from build123d import *

# Parameters (mm, degrees)
F0_W      = 39.5
F0_H      = 15
F1_DEPTH  = 5
F2_W      = 1.5
F2_H      = 15
F3_DEPTH  = 15
F5_W      = 1.5
F5_H      = 15
F6_DEPTH  = 15
F7_DEPTH  = 12.95
F9_W      = 0.5
F9_H      = 1.5
F10_DEPTH = 15
F9_W_2    = 1.5
F9_H_2    = 2.05
F9_H_3    = 2.0491243154
F11_DEPTH = 15
F13_DEPTH = 15
F14_W     = 0.5
F14_H     = 1.45
F15_DEPTH = 15


# Not quite as in the source:
# - the program builds the solid bodies; features that only make, move or delete a surface that nothing else refers to are left out


with BuildPart() as f1:
    # F0 (on Top) → F1 (new body)
    with BuildSketch(Plane.XY):
        Rectangle(F0_W, F0_H)
    extrude(amount=F1_DEPTH)

    # F2 (on face) → F3 (join)
    with BuildSketch(Plane.XY.offset(5)):
        with Locations((-19, 0)):
            Rectangle(F2_W, F2_H)
        with Locations((-9.5, 0)):
            Rectangle(F2_W, F2_H)
        Rectangle(F2_W, F2_H)
        with Locations((9.5, 0)):
            Rectangle(F2_W, F2_H)
        with Locations((19, 0)):
            Rectangle(F2_W, F2_H)
    extrude(amount=F3_DEPTH)

    # F5 (on face) → F6 (join)
    with BuildSketch(Plane(origin=(0, 0, 0), x_dir=(1, 0, 0), z_dir=(0, 0, -1))):
        with Locations((-19, 0)):
            Rectangle(F5_W, F5_H)
        with Locations((19, 0)):
            Rectangle(F5_W, F5_H)
    extrude(amount=F6_DEPTH)

    # F5 (on face) → F7 (join)
    with BuildSketch(Plane(origin=(0, 0, 0), x_dir=(1, 0, 0), z_dir=(0, 0, -1))):
        with Locations((-9.5, 0)):
            Rectangle(F5_W, F5_H)
        Rectangle(F5_W, F5_H)
        with Locations((9.5, 0)):
            Rectangle(F5_W, F5_H)
    extrude(amount=F7_DEPTH)

    # F9 (on face) → F10 (cut)
    with BuildSketch(Plane(origin=(0, 7.5, 0), x_dir=(-1, 0, 0), z_dir=(0, 1, 0))):
        with Locations((18.5, 18.75)):
            Rectangle(F9_W, F9_H)
        with Locations((-18.5, 18.75)):
            Rectangle(F9_W, F9_H)
    extrude(amount=-F10_DEPTH, mode=Mode.SUBTRACT)

    # F9 (on face) → F11 (cut)
    with BuildSketch(Plane(origin=(0, 7.5, 0), x_dir=(-1, 0, 0), z_dir=(0, 1, 0))):
        with Locations((-9.5, 18.975)):
            Rectangle(F9_W_2, F9_H_2)
        with Locations((0, 18.9754378423)):
            Rectangle(F9_W_2, F9_H_3)
        with Locations((9.5, 18.9754378423)):
            Rectangle(F9_W_2, F9_H_3)
    extrude(amount=-F11_DEPTH, mode=Mode.SUBTRACT)

    # F12 (on face) → F13 (join)
    with BuildSketch(Plane.XZ.offset(7.5)):
        Polygon((-18.25, 19.5), (-18.75, 19.5), (-18.75, 18.05), (18.7, 18.05), (18.7, 19.5), (18.25, 19.5), align=None)
    extrude(amount=-F13_DEPTH)

    # F14 (on face) → F15 (cut)
    with BuildSketch(Plane.XZ.offset(7.5)):
        with Locations((18.5, -13.775)):
            Rectangle(F14_W, F14_H)
        with Locations((-18.5, -13.775)):
            Rectangle(F14_W, F14_H)
    extrude(amount=-F15_DEPTH, mode=Mode.SUBTRACT)


solid = f1.part
The listing builds one solid part. Answer for the finished solid, in the listing's coordinates (mm). A direction names the side the tool comes from. Give positions to 0.01 mm unless a question says otherwise; leave off trailing zeros. Write each loop counter-clockwise with the first axis right and the second up, starting at its lowest first coordinate (ties: lowest second). Pieces come first, ordered by that corner, then holes. Notation, with made-up numbers: (-9, -2) - (47, -2) arc R21 ccw to (47, 25) - close; hole circle Ø10 at (-24, 11). An arc over 180 degrees is marked (long way). Use a Markdown table: item, result.
1. Each of these flat-tipped pins is pushed along its axis until it touches: P1, Ø4, axis at x = -6, y = 1.5, coming from the +Z side; P2, Ø2, axis at x = -4, y = 0.5, coming from the -Z side. Where does it stop, or does it pass through?
Values follow:
| item | result |
|---|---|
| P1 | stops at z = 19.5 |
| P2 | stops at z = 0 |
2. A tool of negligible diameter and unlimited length cuts with its end or side. For faces 5 (the flat face through (18.75, 0, -14)), 6 (the flat face through (0, 0, 19.5)), 7 (the flat face through (-8.75, 0, -6)), from which of +Z, -Z, +X, -X, +Y, -Y can it reach the whole face along a straight path? Write none if from no direction.
Values follow:
| item | result |
|---|---|
| face 5 | +Y, -Y |
| face 6 | +Z, +Y, -Y |
| face 7 | -Z, +Y, -Y |
3. For a pull along Z with two mould halves and no side action, classify faces 1 (the flat face through (14, 0, 5)), 2 (the flat face through (0, -7.5, 7)), 3 (the flat face through (-8.75, 0, 11)), 4 (the flat face through (19, 0, -15)) as released by +Z, released by -Z, zero draft, split by the parting line, or undercut.
Values follow:
| item | result |
|---|---|
| face 1 | undercut |
| face 2 | zero draft |
| face 3 | undercut |
| face 4 | released by -Z |
4. Section A-A on z = -2.5 is taken. Write down the section's boundary in (x, y).
Values follow:
| item | result |
|---|---|
| outline | (-19.75, -7.5) - (-18.25, -7.5) - (-18.25, 7.5) - (-19.75, 7.5) - close; (-10.25, -7.5) - (-8.75, -7.5) - (-8.75, 7.5) - (-10.25, 7.5) - close; (-0.75, -7.5) - (0.75, -7.5) - (0.75, 7.5) - (-0.75, 7.5) - close; (8.75, -7.5) - (10.25, -7.5) - (10.25, 7.5) - (8.75, 7.5) - close; (18.25, -7.5) - (19.75, -7.5) - (19.75, 7.5) - (18.25, 7.5) - close |
5. Section B-B on x = 9.5 is taken. Write down the section's boundary in (y, z).
Values follow:
| item | result |
|---|---|
| outline | (-7.5, -12.95) - (7.5, -12.95) - (7.5, 17.95) - (-7.5, 17.95) - close; (-7.5, 18.05) - (7.5, 18.05) - (7.5, 19.5) - (-7.5, 19.5) - close |
6. Section C-C on x = -13 is taken. Write down the section's boundary in (y, z), plus the area to 4 significant figures.
Values follow:
| item | result |
|---|---|
| outline | (-7.5, 0) - (7.5, 0) - (7.5, 5) - (-7.5, 5) - close; (-7.5, 18.05) - (7.5, 18.05) - (7.5, 19.5) - (-7.5, 19.5) - close |
| area | 96.75 mm² |
7. Find the intervals of material crossed by probe 1 along X at (y, z) = (6.75, -4); probe 2 along Z at (x, y) = (-3, 3.25), in increasing order. Write a range as from..to.
Values follow:
| item | result |
|---|---|
| probe 1 | x = -19.75..-18.25, -10.25..-8.75, -0.75..0.75, 8.75..10.25, 18.25..19.75 |
| probe 2 | z = 0..5, 18.05..19.5 |
